CAD build for the part. Positions are in the model's coordinates, mm. Face numbers are marked on the shaded views. A direction names the side the tool comes from. Give positions to 0.01 mm unless a question says otherwise; leave off trailing zeros. Loops run counter-clockwise (first coordinate to the right, second up) from the corner with the lowest first, then second, coordinate; pieces in that order, holes last.
Autodesk Inventor part; units mm, degrees
ref_plane "YZ Plane" through (0, 0, 0) normal (1, 0, 0) x (0, 1, 0)
ref_plane "XZ Plane" through (0, 0, 0) normal (0, 1, 0) x (-1, 0, 0)
ref_plane "XY Plane" through (0, 0, 0) normal (0, 0, 1) x (1, 0, 0)
sketch "Sketch2" plane through (0, 0, 0) normal (0, 0, 1) x (1, 0, 0)
  line L0 (5, 5) -> (10, 5)
  line L1 (10, 5) -> (10, 0)
  line L2 (10, 0) -> (5, 0)
  line L3 (5, 0) -> (5, 5)
  line L4 (0, 5) -> (40, 5)
  line L5 (40, 5) -> (40, 30)
  line L6 (40, 30) -> (0, 30)
  line L7 (0, 30) -> (0, 5)
  line L8 (20, 5) -> (20, 0)
  line L9 (20, 0) -> (15, 0)
  line L10 (15, 0) -> (15, 5)
  line L11 (30, 5) -> (30, 0)
  line L12 (30, 0) -> (25, 0)
  line L13 (25, 0) -> (25, 5)
  line L14 (40, 20) -> (40, 15)
  line L15 (40, 10) -> (40, 5)
  line L16 (40, 30) -> (40, 5)
  line L17 (35, 25) -> (40, 25)
  line L18 (40, 25) -> (40, 20)
  line L19 (40, 20) -> (35, 20)
  line L20 (35, 20) -> (35, 25)
  line L21 (35, 15) -> (40, 15)
  line L22 (40, 15) -> (40, 10)
  line L23 (40, 10) -> (35, 10)
  line L24 (35, 10) -> (35, 15)
  line L25 (10, 30) -> (5, 30)
  line L26 (20, 30) -> (15, 30)
  line L27 (30, 30) -> (25, 30)
  line L28 (40, 30) -> (35, 30)
  line L29 (0, 35) -> (5, 35)
  line L30 (5, 35) -> (5, 30)
  line L31 (5, 30) -> (0, 30)
  line L32 (0, 30) -> (0, 35)
  line L33 (15, 35) -> (15, 30)
  line L34 (15, 30) -> (10, 30)
  line L35 (10, 30) -> (10, 35)
  line L36 (10, 35) -> (15, 35)
  line L37 (25, 35) -> (25, 30)
  line L38 (25, 30) -> (20, 30)
  line L39 (20, 30) -> (20, 35)
  line L40 (20, 35) -> (25, 35)
  line L41 (35, 35) -> (35, 30)
  line L42 (35, 30) -> (30, 30)
  line L43 (30, 30) -> (30, 35)
  line L44 (30, 35) -> (35, 35)
  line L45 (40, 0) -> (35, 0)
  line L46 (35, 0) -> (35, 35)
  line L47 (35, 35) -> (40, 35)
  line L48 (40, 35) -> (40, 0)
  point P0 (0, 0)
  point P1 (35, 5)
  dimension "d105" = 10
  dimension "d110" = 40
  dimension "d115" = 10
extrude "Extrusion3" add sketch "Sketch2" along normal blind 5 contours L4 L7 L6 L46 L20 L24 L0 | L0 L1 L2 L3 | L4 L8 L9 L10 | L32 L29 L30 L6 | L4 L11 L12 L13 | L35 L36 L33 L6 | L39 L40 L37 L6 | L24 L21 L5 L23 | L43 L44 L41 L6 | L20 L17 L5 L19 | L41 L47 L48 L6
properties part number "backside"
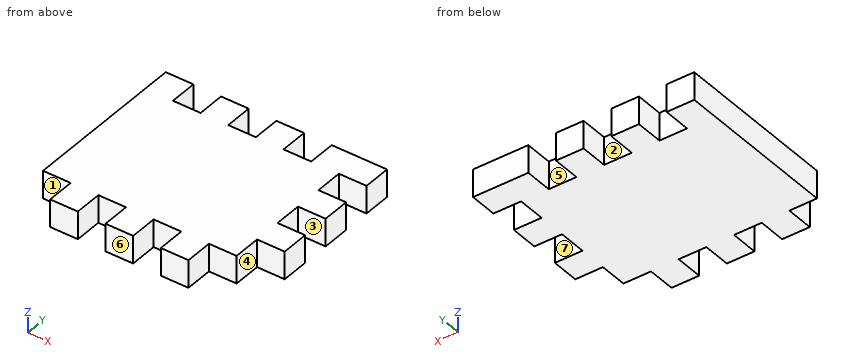
1. Tool access for the marked faces 1, 2, 3 and 4: list every direction of +Z, -Z, +X, -X, +Y, -Y with a clear straight run to the whole face (end or side of a thin tool).
Responses:
face 1: +Z, -Z, -X, -Y
face 2: +Z, -Z, +Y
face 3: +Z, -Z, +X
face 4: +Z, -Z, +X, -Y
2. Saw through at A-A, the plane y = 32.5. List the corners of the cut face in (x, z), and give its area (3 significant figures).
Responses:
outline: (0, 0) - (5, 0) - (5, 5) - (0, 5) - close; (10, 0) - (15, 0) - (15, 5) - (10, 5) - close; (20, 0) - (25, 0) - (25, 5) - (20, 5) - close; (30, 0) - (40, 0) - (40, 5) - (30, 5) - close
area: 125 mm2
3. Drop flat-ended pins along their axis: pin 1 (3 mm diameter, centred on y = 15.5, z = 3, fed in from +X); pin 2 (2.5 mm diameter, centred on x = 38, z = 2.5, fed in from -Y); pin 3 (1.5 mm diameter, centred on x = 11.5, z = 1.5, fed in from -Y); pin 4 (1.5 mm diameter, centred on y = 17, z = 2, fed in from +X). Give the stop position or say it passes through.
Responses:
pin 1: stops at x = 40
pin 2: stops at y = 10
pin 3: stops at y = 5
pin 4: stops at x = 35
4. Saw through at C-C, the plane y = 16. List the corners of the cut face in (x, z).
Responses:
outline: (0, 0) - (35, 0) - (35, 5) - (0, 5) - close
5. Probe line 1 along Y through (x, z) = (37, 2.45); line 2 along X through (y, z) = (28, 3.75); line 3 along Y through (x, z) = (24, 4.5). List the from-to ranges inside material, lowest first.
Responses:
line 1: y = 10 to 15, 20 to 25, 30 to 35
line 2: x = 0 to 35
line 3: y = 5 to 35
6. Saw through at B-B, the plane x = 4. List the corners of the cut face in (y, z), and give its area (3 significant figures).
Responses:
outline: (5, 0) - (35, 0) - (35, 5) - (5, 5) - close
area: 150 mm2
7. Pull direction Y, two halves, no side cores. Call the marked faces 5, 6 and 7: released by +Y, released by -Y, zero draft, split by the parting line, or undercut.
Responses:
face 5: released by +Y
face 6: released by -Y
face 7: undercut
